from build123d import *

# Parameters (mm, degrees)
F1_DEPTH = 63.5
F2_R     = 4.7625
F3_DEPTH = 9.525


with BuildPart() as f1:
    # F0 (on Top) → F1 (new body, symmetric)
    with BuildSketch(Plane.XY):
        Polygon((-1663.7, 0), (-1663.7, -9.525), (-1473.2, -9.525), (-1473.2, 0), (-1422.4, 0), (-1422.4, -9.525), (-723.9, -9.525), (-723.9, 0), (-673.1, 0), (-673.1, -9.525), (-50.8, -9.525), (-50.8, 0), (0, 0), (0, 9.525), (-1696.990768, 9.525), (-1693.045384, 0), align=None)
    extrude(amount=F1_DEPTH, both=True)

    # F2 (on Right) → F3 (join)
    with BuildSketch(Plane.YZ):
        Circle(F2_R)
    extrude(amount=F3_DEPTH)


solid = f1.part
Verification items for the finished model (mm, model axes). A direction names the side the tool comes from. Coordinates: 2 decimals unless noted, no trailing zeros. Write each loop counter-clockwise with the first axis right and the second up, starting at its lowest first coordinate (ties: lowest second). Pieces come first, ordered by that corner, then holes. Notation, with made-up numbers: M 78.5,-15 L 107.5,-15 A20 ccw 107.5,18 Z; hole C 50.5,-3 d5. An arc over 180 degrees is marked long. Use a Markdown table: item, result.
Q1. Go/stop test with flat-tipped pins: P1, Ø2, axis at y = 4.5, z = -6.5, coming from the -X side; P2, Ø10.5, axis at y = -2.5, z = 30.5, coming from the +X side; P3, Ø9, axis at x = -1674.5, z = -9.5, coming from the -Y side. Record where each tip stops, or that it passes through.
Reply:
| item | result |
|---|---|
| P1 | stops at x = -1695.32 |
| P2 | stops at x = 0 |
| P3 | stops at y = 0 |
Q2. Set-up check for faces 3 (the face through (-1448, 0, 1)), 4 (the face through (-1679, 0, 1)), 5 (the face through (-1570, -9.525, 1)): record each of +Z, -Z, +X, -X, +Y, -Y from which the full face is reachable in a straight line by a thin tool's end or side.
Reply:
| item | result |
|---|---|
| face 3 | +Z, -Z, -Y |
| face 4 | +Z, -Z, -X, -Y |
| face 5 | +Z, -Z, +X, -X, -Y |
Q3. Draft check along X on faces 1 (the face through (-837, 9.525, 1)), 2 (the face through (-699, 0, 1)). Enter one of: +X half, -X half, draft (parallel to the pull), parting line (faces both ways), or undercut.
Reply:
| item | result |
|---|---|
| face 1 | draft |
| face 2 | undercut |
Q4. Sectioned sample at A-A, the plane z = -23. Record the boundary of the cut face in (x, y) (3 decimals).
Reply:
| item | result |
|---|---|
| outline | M -1696.991,9.525 L -1693.045,0 L -1663.7,0 L -1663.7,-9.525 L -1473.2,-9.525 L -1473.2,0 L -1422.4,0 L -1422.4,-9.525 L -723.9,-9.525 L -723.9,0 L -673.1,0 L -673.1,-9.525 L -50.8,-9.525 L -50.8,0 L 0,0 L 0,9.525 Z |
Q5. Thickness scan on line 1 (X direction, y = -7.5, z = -29.5); line 2 (X direction, y = 5.75, z = -49.5); line 3 (X direction, y = 8.5, z = 53.5). Record the ranges inside material, lowest first.
Reply:
| item | result |
|---|---|
| line 1 | x = -1663.7 to -1473.2, -1422.4 to -723.9, -673.1 to -50.8 |
| line 2 | x = -1695.43 to 0 |
| line 3 | x = -1696.57 to 0 |
